```python
from build123d import *

# Parameters (mm, degrees)
F0_W     = 914.4
F0_H     = 609.6
F1_DEPTH = 25.4
F2_R     = 12.7
F3_DEPTH = 57.15
F5_D     = 12.7


with BuildPart() as f1:
    # F0 (on Right) → F1 (new body)
    with BuildSketch(Plane.YZ):
        Rectangle(F0_W, F0_H)
    extrude(amount=F1_DEPTH)

    # F2 (on face) → F3 (join)
    with BuildSketch(Plane.YZ.offset(25.4)):
        Circle(F2_R)
    extrude(amount=F3_DEPTH)

    # F5 (through all)
    with Locations(Plane.YZ.offset(25.4)):
        with Locations((-101.6, -158.75), (101.6, -158.75), (101.6, -222.25), (-101.6, -222.25)):
            Hole(F5_D / 2)


solid = f1.part
```
Source: CAD feature listing. Evaluate the final solid. Frame: model axes, mm. A direction names the side the tool comes from. Round coordinates to 2 decimals unless told otherwise and drop trailing zeros. Loops run counter-clockwise (first coordinate to the right, second up) from the corner with the lowest first, then second, coordinate; pieces in that order, holes last. Notation, with made-up numbers: M 15,-8 L 67,-8 A36 cw 67,29 Z; hole C 26.25,29 d11. An arc over 180 degrees is marked long. Use a Markdown table: item, result. Add a question column.
1. Section query B-B on x = 52.5. Return the cut outline in (y, z), then the cut area to 3 significant figures.
2. Section query C-C on y = 24. Return the cut outline in (x, z).
3. Reachability of faces 1 (the flat face through (13, -6, 304.8)), 2 (the cylindrical face through (53.57, -2.75, -12.4)) from +Z, -Z, +X, -X, +Y, -Y: full face, straight path, thin tool, end or side. Return the list, or none.
4. Section query D-D on z = 123. Return the cut outline in (x, y).
5. Contact query for flat-ended pins moving along their axis: P1, Ø14.5, axis at y = 101.6, z = -222.25, coming from the -X side; P2, Ø5, axis at y = -26, z = -228.5, coming from the +X side; P3, Ø8, axis at x = 30, z = 145.5, coming from the -Y side; P4, Ø4, axis at x = 73, z = 4, coming from the -Y side. Output: stop coordinate, or through.
6. Section query A-A on z = 0. Return the cut outline in (x, y).
7. Line query: line 1 (Y direction, x = 18, z = -158); line 2 (Z direction, x = 9.5, y = -101.6); line 3 (X direction, y = -268, z = -177). Output: solid intervals per line, ascending.
Reported:
| question | item | result |
|---|---|---|
| 1 | outline | C 0,0 d25.4 |
| 1 | area | 507 mm² |
| 2 | outline | M 0,-304.8 L 25.4,-304.8 L 25.4,304.8 L 0,304.8 Z |
| 3 | face 1 | +Z, +X, -X, +Y, -Y |
| 3 | face 2 | +X |
| 4 | outline | M 0,-457.2 L 25.4,-457.2 L 25.4,457.2 L 0,457.2 Z |
| 5 | P1 | stops at x = 0 |
| 5 | P2 | stops at x = 25.4 |
| 5 | P3 | passes through |
| 5 | P4 | stops at y = -12.54 |
| 6 | outline | M 0,-457.2 L 25.4,-457.2 L 25.4,-12.7 L 82.55,-12.7 L 82.55,12.7 L 25.4,12.7 L 25.4,457.2 L 0,457.2 Z |
| 7 | line 1 | y = -457.2 to -107.91, -95.29 to 95.29, 107.91 to 457.2 |
| 7 | line 2 | z = -304.8 to -228.6, -215.9 to -165.1, -152.4 to 304.8 |
| 7 | line 3 | x = 0 to 25.4 |
